Here's how the part is built. I have some questions about the finished solid (model axes, mm). Coordinates: 2 decimals unless noted, no trailing zeros. Write each loop counter-clockwise with the first axis right and the second up, starting at its lowest first coordinate (ties: lowest second). Pieces come first, ordered by that corner, then holes. Notation, with made-up numbers: (7, 44) - (45, 44) arc R13 cw to (45, 52) - close; hole circle Ø9 at (28.5, 56). An arc over 180 degrees is marked (long way). Answer in a Markdown table with one row per item. Add a question column.
Item 1: Imagine slicing it at C-C (z = -73.5). Please give me the cut outline in (x, y).
Item 2: Imagine slicing it at A-A (z = -42.5). Please give me the cut outline in (x, y).
Item 3: If I drill on probe 1 along X at (y, z) = (3.55, -14); probe 2 along Z at (x, y) = (-2.5, 1.95); probe 3 along Z at (x, y) = (-25, 0.65), over which ranges is the centre line in solid material (lowest first)? Write a range as from..to.
Item 4: We'd pull the mould along X, two halves only. Please class faces 1 (the face through (-70, 2, -40)), 2 (the face through (-57.82, 1.97, -43.67)), 3 (the face through (-30, 2, 0)): +X half, -X half, draft (parallel to the pull), parting line (faces both ways), or undercut.
Item 5: Imagine slicing it at B-B (x = -34.5). Please give me the cut outline in (y, z), plus the area to 3 significant figures.
Item 6: I'm going to push a flat-ended pin straight in: pin 1 (1.5 mm diameter, centred on y = 2, z = -72, fed in from -X). Where does the tip first touch, or does it pass through?
Item 7: Imagine slicing it at D-D (y = 2.8). State how many separate pieces and enclosed holes the cut face has, plus the area to 3 significant figures.
Autodesk Inventor part; units mm, degrees
ref_plane "YZ Plane" through (0, 0, 0) normal (1, 0, 0) x (0, 1, 0)
ref_plane "XZ Plane" through (0, 0, 0) normal (0, 1, 0) x (-1, 0, 0)
ref_plane "XY Plane" through (0, 0, 0) normal (0, 0, 1) x (1, 0, 0)
sketch "Sketch1" plane through (0, 0, 0) normal (0, 1, 0) x (-1, 0, 0)
  line L0 (0, 0) -> (60, 0)
  line L1 (60, 0) -> (60, -81)
  line L2 (60, -81) -> (0, -81)
  line L3 (0, -81) -> (0, 0)
  line L4 (45, -21.6284) -> (15, -21.6284) construction
  line L5 (45, -81) -> (45, 0) construction
  line L6 (15, 0) -> (15, -81) construction
  circle A0 centre (40, -73.5) radius 1.5
  circle A1 centre (40, -7.5) radius 1.5
  circle A2 centre (20, -7.5) radius 1.5
  circle A3 centre (20, -73.5) radius 1.5
  line L7 (60, -40.5) -> (0, -40.5) construction
  line L8 (30, 0) -> (30, -81) construction
  circle A4 centre (30, -40.5) radius 24
  circle A5 centre (30, -40.5) radius 27.5
  circle A6 centre (57.1293, -36) radius 1.5
  circle A7 centre (57.1293, -45) radius 1.5
  circle A8 centre (25.5, -13.3707) radius 1.5
  circle A9 centre (34.5, -13.3707) radius 1.5
  circle A10 centre (2.8707, -45) radius 1.5
  circle A11 centre (2.8707, -36) radius 1.5
  circle A12 centre (34.5, -67.6293) radius 1.5
  circle A13 centre (25.5, -67.6293) radius 1.5
  circle A14 centre (30, -40.5) radius 40 construction
  arc A15 (60, -81) -> (60, 0) centre (-17.0125, -40.5) ccw
  circle A16 centre (30, -40.5) radius 36.28 construction
  circle A17 centre (65.9998, -36) radius 1.5
  circle A18 centre (65.9998, -45) radius 1.5
  circle A19 centre (-5.9998, -45) radius 1.5
  circle A20 centre (-5.9998, -36) radius 1.5
  arc A21 (0, 0) -> (0, -81) centre (77.0125, -40.5) ccw
  line L9 (30, -40.5) -> (-3.3536, -73.8536) construction
  circle A22 centre (1.7157, -68.7843) radius 1.5
  circle A23 centre (11.8404, -76.1403) radius 1.5
  circle A24 centre (23.7426, -80.0075) radius 1.5
  circle A25 centre (36.2574, -80.0075) radius 1.5
  circle A26 centre (48.1596, -76.1403) radius 1.5
  circle A27 centre (58.2843, -68.7843) radius 1.5
  circle A28 centre (65.6403, -58.6596) radius 1.5
  circle A29 centre (69.5075, -46.7574) radius 1.5
  circle A30 centre (69.5075, -34.2426) radius 1.5
  circle A31 centre (65.6403, -22.3404) radius 1.5
  circle A32 centre (58.2843, -12.2157) radius 1.5
  circle A33 centre (48.1596, -4.8597) radius 1.5
  circle A34 centre (36.2574, -0.9925) radius 1.5
  circle A35 centre (23.7426, -0.9925) radius 1.5
  circle A36 centre (11.8404, -4.8597) radius 1.5
  circle A37 centre (1.7157, -12.2157) radius 1.5
  circle A38 centre (-5.6403, -22.3404) radius 1.5
  circle A39 centre (-9.5075, -34.2426) radius 1.5
  circle A40 centre (-9.5075, -46.7574) radius 1.5
  circle A41 centre (-5.6403, -58.6596) radius 1.5
  circle A42 centre (48.1596, -68.7843) radius 1.5
  circle A43 centre (48.1596, -12.2157) radius 1.5
  circle A44 centre (11.8404, -12.2157) radius 1.5
  circle A45 centre (11.8404, -68.7843) radius 1.5
  point P0 (30, -21.6284)
  dimension "d31" = 80
  dimension "width" = 60
  dimension "d1" = 81
  dimension "fixed" = 3
  dimension "d6" = 7.5
  dimension "d7" = 5
  dimension "d8" = 30
  dimension "d9" = 3
  dimension "d10" = 7.5
  dimension "d11" = 5
  dimension "d12" = 3
  dimension "d13" = 3
  dimension "d14" = 5
  dimension "d19" = 48
  dimension "d20" = 55
  dimension "d21" = 3
  dimension "d22" = 4.5
  dimension "d23" = 3
  dimension "d24" = 4.5
  dimension "d27" = 360
  dimension "d32" = 72.56
  dimension "d33" = 3
  dimension "d34" = 3
  dimension "d37" = 360
  dimension "d39" = 45
  dimension "d40" = 3
  dimension "d43" = 360
  dimension "d47" = 3
  dimension "d48" = 3
  dimension "d49" = 3
  dimension "d50" = 3
extrude "Extrusion1" add sketch "Sketch1" along normal blind 4 contours L0 A35 A34 L1 L2 A25 A24 L3 | L3 A21 A40 A39 | L0 A35 | A39 A21 | A24 L2 | A21 A40 | L0 A34 | A25 L2 | A15 A30 A29 L1 | A15 A30 | A29 A15 | A4 | A5 A7 A12 A13 A10 A11 A8 A9 A6 | A6 A5 | A5 A6 | A7 A5 | A5 A7 | A9 A5 | A5 A9 | A12 A5 | A5 A12 | A8 A5 | A5 A8 | A13 A5 | A5 A13 | A11 A5 | A5 A11 | A10 A5 | A5 A10 | A22 | A23 | A26 | A27 | A28 | A31 | A32 | A33 | A36 | A37 | A38 | A41 | A42 | A43 | A44 | A45 picked at (23.6828, -0.8272) picked at (-9.1838, -34.2299) picked at (24.0268, -80.2578) picked at (-9.1838, -46.7701) picked at (35.7864, -0.994) picked at (35.8837, -79.4355) picked at (69.1851, -34.2659) picked at (69.1851, -46.7341)
extrude "Extrusion2" cut sketch "Sketch1" along normal blind 10 contours A4 | A6 A5 | A5 A6 | A7 A5 | A5 A7 | A9 A5 | A5 A9 | A12 A5 | A5 A12 | A8 A5 | A5 A8 | A13 A5 | A5 A13 | A11 A5 | A5 A11 | A10 A5 | A5 A10
extrude "Extrusion3" cut sketch "Sketch1" along normal blind 10 contours A22 | A23 | A26 | A27 | A28 | A31 | A32 | A33 | A36 | A37 | A38 | A41 | A42 | A43 | A44 | A45
equation "\"d8\" = 0.5 * width"
equation "\"d9\" = fixed"
equation "\"d12\" = fixed"
equation "\"d13\" = fixed"
equation "\"d23\" = fixed"
equation "\"d33\" = fixed"
equation "\"d34\" = fixed"
equation "\"d40\" = fixed"
equation "\"d47\" = fixed"
equation "\"d48\" = fixed"
equation "\"d49\" = fixed"
equation "\"d50\" = fixed"
properties part number "payload-plateV2"
Here are the results:
| question | item | result |
|---|---|---|
| 1 | outline | (-63.5, 0) - (-41.5, 0) - (-41.5, 4) - (-63.5, 4) - close; (-38.5, 0) - (-21.5, 0) - (-21.5, 4) - (-38.5, 4) - close; (-18.5, 0) - (3.5, 0) - (3.5, 4) - (-18.5, 4) - close |
| 2 | outline | (-69.98, 0) - (-53.92, 0) - (-53.92, 4) - (-69.98, 4) - close; (-6.08, 0) - (9.98, 0) - (9.98, 4) - (-6.08, 4) - close |
| 3 | probe 1 | x = -65.87..-35.86, -33.14..-26.86, -24.14..5.87 |
| 3 | probe 2 | z = -81..-70.06, -67.51..-46.45, -43.55..-37.45, -34.55..-13.49, -10.94..0 |
| 3 | probe 3 | z = -81..-69.04, -66.22..-63.97, -17.03..-14.78, -11.96..0 |
| 4 | face 1 | -X half |
| 4 | face 2 | undercut |
| 4 | face 3 | draft |
| 5 | outline | (0, -81) - (4, -81) - (4, -69.13) - (0, -69.13) - close; (0, -66.13) - (4, -66.13) - (4, -64.07) - (0, -64.07) - close; (0, -16.93) - (4, -16.93) - (4, -14.87) - (0, -14.87) - close; (0, -11.87) - (4, -11.87) - (4, 0) - (0, 0) - close |
| 5 | area | 111 mm2 |
| 6 | pin 1 | stops at x = -64.39 |
| 7 | separate pieces | 1 |
| 7 | enclosed holes | 33 |
| 7 | area | 3,920 mm2 |
